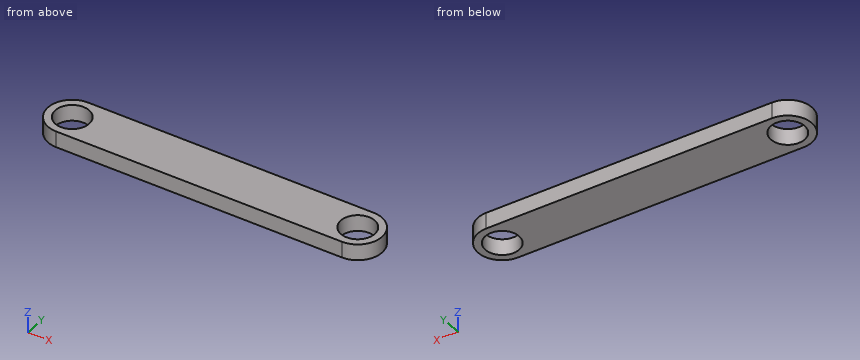
from build123d import *

# Parameters (mm, degrees)
SKETCH_1_R      = 4.2
EXTRUDE_1_DEPTH = 4


with BuildPart() as part:
    # 草图1 → 凸台-拉伸1 (new body)
    with BuildSketch(Plane(origin=(0, 0, 0), x_dir=(-1, 0, 0), z_dir=(0, 0, -1))):
        with BuildLine():
            Line((20, 6), (-50, 6))
            ThreePointArc((-50, 6), (-56, 0), (-50, -6))
            Line((-50, -6), (20, -6))
            ThreePointArc((20, -6), (26, 0), (20, 6))
        make_face()
        with Locations(Location((20, 0, 0), (0, 0, 180))):
            Circle(SKETCH_1_R, mode=Mode.SUBTRACT)
        with Locations(Location((-50, 0, 0), (0, 0, 180))):
            Circle(SKETCH_1_R, mode=Mode.SUBTRACT)
    extrude(amount=-EXTRUDE_1_DEPTH)


solid = part.part
Input: part model. Units: mm. Frame: model coordinates. Give positions to 0.01 mm unless a question says otherwise; leave off trailing zeros. Order: outer loops, then holes, each group sorted by start corner. A loop starts at its lowest first (then second) coordinate and runs counter-clockwise, first axis right, second up. Notation, with made-up numbers: (-11.75, 83) - (6.25, 83) arc R18 cw to (6.25, 101) - close; hole circle Ø9 at (-28.5, -25.75). An arc over 180 degrees is marked (long way). Write each question's results on one line, items separated by ' | '.
Item 1: Material intervals for line 1 along Y through (x, z) = (-20, 2.5); line 2 along X through (y, z) = (0.25, 2.4); line 3 along X through (y, z) = (2.5, 0.55), sorted ascending.
A:
line 1: y = -6 to -4.2, 4.2 to 6 | line 2: x = -25.99 to -24.19, -15.81 to 45.81, 54.19 to 55.99 | line 3: x = -25.45 to -23.37, -16.63 to 46.63, 53.37 to 55.45
Item 2: Section A-A (y = 0). Return loops of the section in (x, z).
A:
outline: (-26, 0) - (-24.2, 0) - (-24.2, 4) - (-26, 4) - close; (-15.8, 0) - (45.8, 0) - (45.8, 4) - (-15.8, 4) - close; (54.2, 0) - (56, 0) - (56, 4) - (54.2, 4) - close
Item 3: Section B-B (z = 2.45). Return loops of the section in (x, y), and give its area (3 significant figures).
A:
outline: (-20, -6) - (50, -6) arc R6 ccw to (50, 6) - (-20, 6) arc R6 ccw to start; hole circle Ø8.4 at (-20, 0); hole circle Ø8.4 at (50, 0) | area: 842 mm^2
